Job drawing, mm, ordinate dimensions from the low corner. One solid piece. Give positions to 0.01 mm unless a question says otherwise; leave off trailing zeros. Write each loop counter-clockwise with the first axis right and the second up, starting at its lowest first coordinate (ties: lowest second). Pieces come first, ordered by that corner, then holes. Notation, with made-up numbers: (-3.75, -39.5) - (21.25, -39.5) arc R11 ccw to (21.25, -28.5) - close; hole circle Ø3 at (50, 48). An arc over 180 degrees is marked (long way). Use a Markdown table: item, result. Add a question column.
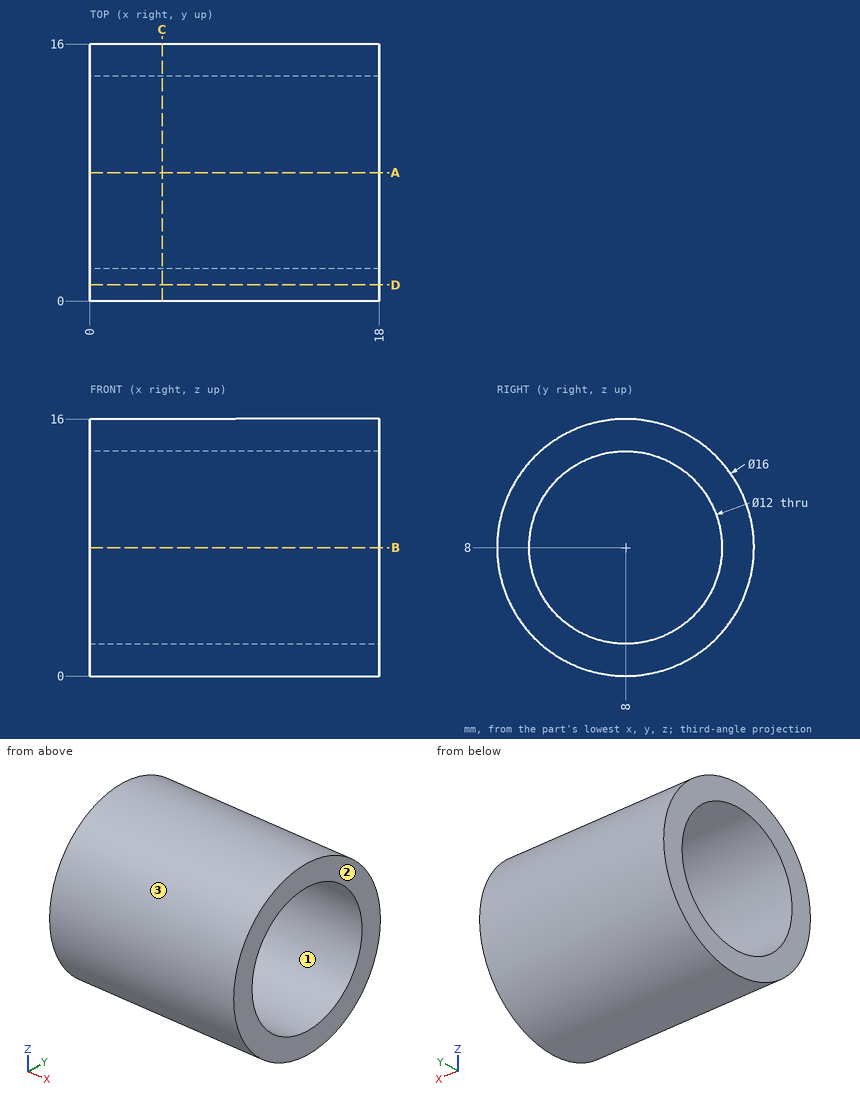
(1) Band-saw the part on D-D (y = 1). Write the cut outline in (x, z).
(2) Band-saw the part on A-A (y = 8). Write the cut outline in (x, z).
(3) Flat gauge pins, fed straight in: pin 1 (1.5 mm diameter, centred on x = 6, y = 9, fed in from +Z); pin 2 (1 mm diameter, centred on x = 3.5, z = 7, fed in from -Y); pin 3 (8 mm diameter, centred on y = 13.5, z = 9, fed in from +X); pin 4 (3 mm diameter, centred on x = 2.5, y = 10.5, fed in from -Z). Where does each tip first touch, or does it go through?
(4) Probe probe 1 along Y at (x, z) = (5.75, 8); probe 2 along Z at (x, y) = (14.75, 8.25); probe 3 along Y at (x, z) = (12, 9.75). List the from-to ranges inside material, lowest first. Write a range as [from, to].
(5) Two-plate mould, pull along Y, no slides. Class the marked faces 1, 2 and 3: +Y half, -Y half, draft (parallel to the pull), parting line (faces both ways), or undercut.
(6) Band-saw the part on C-C (x = 4.5). Write the cut outline in (y, z).
Model answer:
| question | item | result |
|---|---|---|
| 1 | outline | (0, 4.13) - (18, 4.13) - (18, 11.87) - (0, 11.87) - close |
| 2 | outline | (0, 0) - (18, 0) - (18, 2) - (0, 2) - close; (0, 14) - (18, 14) - (18, 16) - (0, 16) - close |
| 3 | pin 1 | stops at z = 16 |
| 3 | pin 2 | stops at y = 0.02 |
| 3 | pin 3 | stops at x = 18 |
| 3 | pin 4 | stops at z = 0.06 |
| 4 | probe 1 | y = [0, 2], [14, 16] |
| 4 | probe 2 | z = [0, 2.01], [13.99, 16] |
| 4 | probe 3 | y = [0.19, 2.26], [13.74, 15.81] |
| 5 | face 1 | undercut |
| 5 | face 2 | draft |
| 5 | face 3 | parting line |
| 6 | outline | circle Ø16 at (8, 8); hole circle Ø12 at (8, 8) |
